Here's how the part is built. I have some questions about the finished solid (model axes, mm). A direction names the side the tool comes from. Round coordinates to 2 decimals unless told otherwise and drop trailing zeros. Loops run counter-clockwise (first coordinate to the right, second up) from the corner with the lowest first, then second, coordinate; pieces in that order, holes last. Notation, with made-up numbers: M 66,-22.75 L 94,-22.75 A9 cw 94,-11.75 Z; hole C -32,-33.5 d3. An arc over 180 degrees is marked long. Write item = value, one per line. Start each with the question number.
from build123d import *

# Parameters (mm, degrees)
SKETCH_1_W          = 68
SKETCH_1_H          = 40
SKETCH_1_R          = 2.5
EXTRUDE_1_DEPTH     = 26
SKETCH_2_R          = 5
CUT_EXTRUDE_1_DEPTH = 76
SKETCH_3_W          = 68
SKETCH_3_H          = 10
CUT_EXTRUDE_2_DEPTH = 5
CHAMFER_1_SIZE      = 5
CHAMFER_2_SIZE      = 5
SKETCH_4_W          = 68
SKETCH_4_H          = 1
CUT_EXTRUDE_3_DEPTH = 9
CHAMFER_3_SIZE      = 1
CHAMFER_4_SIZE      = 1


with BuildPart() as part:
    # Эскиз1 → Бобышка-Вытянуть1 (new body)
    with BuildSketch(Plane(origin=(0, 0, 0), x_dir=(1, 0, 0), z_dir=(0, 1, 0))):
        with Locations((34, 20)):
            Rectangle(SKETCH_1_W, SKETCH_1_H)
        with Locations(Location((11, 34, 0), (0, 0, 90))):
            Circle(SKETCH_1_R, mode=Mode.SUBTRACT)
        with Locations(Location((11, 6, 0), (0, 0, 90))):
            Circle(SKETCH_1_R, mode=Mode.SUBTRACT)
        with Locations(Location((57, 34, 0), (0, 0, 90))):
            Circle(SKETCH_1_R, mode=Mode.SUBTRACT)
        with Locations(Location((57, 6, 0), (0, 0, 90))):
            Circle(SKETCH_1_R, mode=Mode.SUBTRACT)
    extrude(amount=EXTRUDE_1_DEPTH)

    # Эскиз2 → Вырез-Вытянуть1 (cut)
    with BuildSketch(Plane.ZY):
        with Locations((-20, 13)):
            Circle(SKETCH_2_R)
    extrude(amount=-CUT_EXTRUDE_1_DEPTH, mode=Mode.SUBTRACT)

    # Эскиз3 → Вырез-Вытянуть2 (cut)
    with BuildSketch(Plane(origin=(0, 26, 0), x_dir=(1, 0, 0), z_dir=(0, 1, 0))):
        with Locations((34, 35)):
            Rectangle(SKETCH_3_W, SKETCH_3_H)
        with Locations((34, 5)):
            Rectangle(SKETCH_3_W, SKETCH_3_H)
    extrude(amount=-CUT_EXTRUDE_2_DEPTH, mode=Mode.SUBTRACT)

    # Фаска1
    chamfer_1_edges = [part.edges().sort_by_distance(p)[0] for p in [
        (34, 26, -30),
    ]]
    chamfer(chamfer_1_edges, length=CHAMFER_1_SIZE - 0.0001)  # a hair under: the kernel refuses the full size

    # Фаска2
    chamfer_2_edges = [part.edges().sort_by_distance(p)[0] for p in [
        (34, 26, -10),
    ]]
    chamfer(chamfer_2_edges, length=CHAMFER_2_SIZE - 0.0001)  # a hair under: the kernel refuses the full size

    # Эскиз4 → Вырез-Вытянуть3 (cut)
    with BuildSketch(Plane(origin=(0, 21, 0), x_dir=(1, 0, 0), z_dir=(0, 1, 0))):
        with Locations((34, 39.5)):
            Rectangle(SKETCH_4_W, SKETCH_4_H)
        with Locations((34, 0.5)):
            Rectangle(SKETCH_4_W, SKETCH_4_H)
    extrude(amount=-CUT_EXTRUDE_3_DEPTH, mode=Mode.SUBTRACT)

    # Фаска3
    chamfer_3_edges = [part.edges().sort_by_distance(p)[0] for p in [
        (34, 12, -40),
    ]]
    chamfer(chamfer_3_edges, length=CHAMFER_3_SIZE - 0.0001)  # a hair under: the kernel refuses the full size

    # Фаска4
    chamfer_4_edges = [part.edges().sort_by_distance(p)[0] for p in [
        (34, 12, 0),
    ]]
    chamfer(chamfer_4_edges, length=CHAMFER_4_SIZE - 0.0001)  # a hair under: the kernel refuses the full size


solid = part.part
Item 1: I want a section at A-A, the plane y = 13. List the corners of the cut face in (x, z) for me.
Item 2: Please list where these lines run through material, in increasing order: line 1 (Z direction, x = 57, y = 6.75); line 2 (X direction, y = 7.5, z = -34); line 3 (X direction, y = 5.25, z = -5). Write a range as [from, to].
Item 3: I want a section at B-B, the plane x = 57. State how many separate pieces and enclosed holes the cut face has, then the cut area to 3 significant figures.
Item 4: I want a section at C-C, the plane z = -20. List the corners of the cut face in (x, y) for me, then the cut area to 3 significant figures.
Item 5: I want a section at D-D, the plane y = 2. List the corners of the cut face in (x, z) for me.
Item 6: Will these pins go through, and if not, where does the flat tip stop? pin 1 Ø3 at (x, z) = (22.5, -36) entering from +Y; pin 2 Ø10 at (x, z) = (26, -6) entering from +Y; pin 3 Ø4.5 at (x, y) = (31.5, 17.5) entering from +Z.
Item 7: We'd pull the mould along X, two halves only. Please class faces 4 (the flat face through (68, 7, -20)), 5 (the flat face through (34, 5, 0)), 6 (the flat face through (0, 7, -20)), 7 (the cylindrical face through (56.249, 10.353, -8.385)): released by +X, released by -X, zero draft, split by the parting line, or undercut.
Item 8: For faces 1 (the flat face through (34, 5, -40)), 2 (the flat face through (34, 17, -1)), 3 (the flat face through (34, 17, -39)), which set-ups out of +Z, -Z, +X, -X, +Y, -Y let a thin tool reach every point of the face, with its end or its side?
Worked out:
q1.outline = M 0,-39 L 68,-39 L 68,-25 L 0,-25 Z; M 0,-15 L 68,-15 L 68,-1 L 0,-1 Z; hole C 11,-34 d5; hole C 11,-6 d5; hole C 57,-34 d5; hole C 57,-6 d5
q2.line_1 = [-40, -36.5], [-31.5, -8.5], [-3.5, 0]
q2.line_2 = [0, 8.5], [13.5, 54.5], [59.5, 68]
q2.line_3 = [0, 8.71], [13.29, 54.71], [59.29, 68]
q3.separate_pieces = 3
q3.enclosed_holes = 1
q3.area = 607 mm2
q4.outline = M 0,0 L 68,0 L 68,8 L 0,8 Z; M 0,18 L 68,18 L 68,26 L 0,26 Z
q4.area = 1,090 mm2
q5.outline = M 0,-40 L 68,-40 L 68,0 L 0,0 Z; hole C 11,-34 d5; hole C 11,-6 d5; hole C 57,-34 d5; hole C 57,-6 d5
q6.pin_1 = 21
q6.pin_2 = 22
q6.pin_3 = -1
q7.face_4 = released by +X
q7.face_5 = zero draft
q7.face_6 = released by -X
q7.face_7 = undercut
q8.face_1 = -Z, +X, -X, +Y, -Y
q8.face_2 = +Z, +X, -X, +Y
q8.face_3 = -Z, +X, -X, +Y
